Geometry check sheet. Reference: drawing and pictorial views, mm from the part's lowest x, y, z. Give positions to 0.01 mm unless a question says otherwise; leave off trailing zeros. Write each loop counter-clockwise with the first axis right and the second up, starting at its lowest first coordinate (ties: lowest second). Pieces come first, ordered by that corner, then holes. Notation, with made-up numbers: (-29, 24.25) -> (19, 24.25) arc R30 ccw to (19, 63.25) -> close; hole circle Ø11 at (30, 85). An arc over 180 degrees is marked (long way). Use a Markdown table: item, result. Add a question column.
1. Cross-section at B-B (z = 12.5). Enter the section's corners in (x, y).
2. Gauge pin test, flat ends, axial feed: P1, Ø1.5, axis at y = 23.5, z = 13.5, coming from the -X side; P2, Ø1.5, axis at y = 26, z = 4, coming from the -X side; P3, Ø8, axis at x = 14, z = 11.5, coming from the +Y side. Record the tip position at first contact, or that the pin passes through.
3. Release check for a two-part mould opening along X. For the marked faces 1, 2, 3 and 4 record: released by +X, released by -X, zero draft, split by the parting line, or undercut.
4. Scan lines: probe 1 along X at (y, z) = (20.75, 12.5); probe 2 along Z at (x, y) = (17.5, 19.5) (3 decimals); probe 3 along X at (y, z) = (21.75, 19). Record each from-to range of solid material in increasing order. Write a range as [from, to].
5. Cross-section at C-C (y = 25.75). Enter the section's corners in (x, z).
6. Cross-section at A-A (x = 12.5). Enter the section's corners in (y, z).
7. Cross-section at D-D (y = 12.75). Enter the section's corners in (x, z), then the cut area to 3 significant figures.
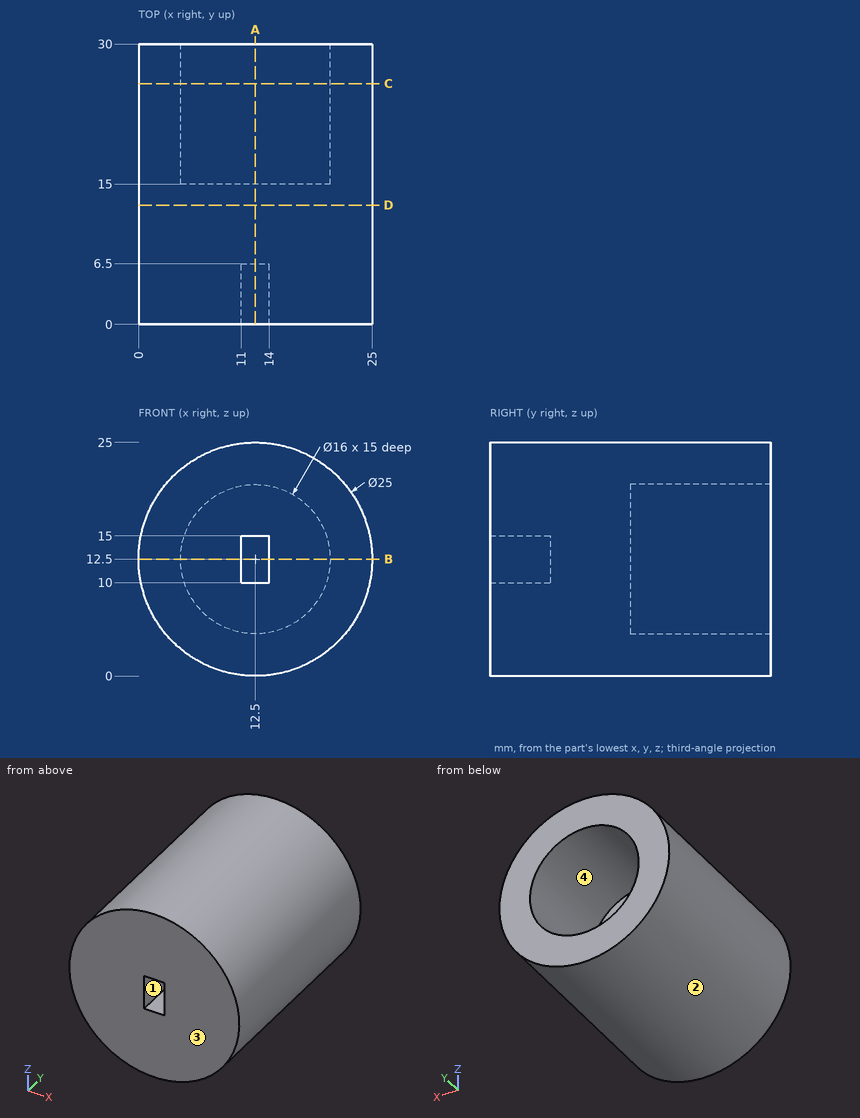
Worked answers:
| question | item | result |
|---|---|---|
| 1 | outline | (0, 0) -> (11, 0) -> (11, 6.5) -> (14, 6.5) -> (14, 0) -> (25, 0) -> (25, 30) -> (20.5, 30) -> (20.5, 15) -> (4.5, 15) -> (4.5, 30) -> (0, 30) -> close |
| 2 | P1 | stops at x = 0 |
| 2 | P2 | stops at x = 2.69 |
| 2 | P3 | stops at y = 15 |
| 3 | face 1 | undercut |
| 3 | face 2 | split by the parting line |
| 3 | face 3 | zero draft |
| 3 | face 4 | undercut |
| 4 | probe 1 | x = [0, 4.5], [20.5, 25] |
| 4 | probe 2 | z = [1.044, 6.255], [18.745, 23.956] |
| 4 | probe 3 | x = [1.82, 7.84], [17.16, 23.18] |
| 5 | outline | circle Ø25 at (12.5, 12.5); hole circle Ø16 at (12.5, 12.5) |
| 6 | outline | (0, 0) -> (30, 0) -> (30, 4.5) -> (15, 4.5) -> (15, 20.5) -> (30, 20.5) -> (30, 25) -> (0, 25) -> (0, 15) -> (6.5, 15) -> (6.5, 10) -> (0, 10) -> close |
| 7 | outline | circle Ø25 at (12.5, 12.5) |
| 7 | area | 491 mm² |
